from build123d import *

# Parameters (mm, degrees)
F0_R     = 11
F0_R_2   = 11.2
F1_DEPTH = 3.6
F2_R     = 11.2
F2_R_2   = 11
F2_R_3   = 9.7
F3_DEPTH = 1.5
F5_R     = 0.9
F6_DEPTH = 5.1
F7_SIZE  = 1


with BuildPart() as f1:
    # F0 (on Top) → F1 (new body)
    with BuildSketch(Plane.XY):
        with BuildLine():
            ThreePointArc((-2.4878611303, 39.4539370079), (-12.6317197215, 28.3151642022), (-5, 15.3256691841))
            Line((-5, 15.3256691841), (-5, 12.539936204))
            ThreePointArc((-5, 12.539936204), (-11.6913429511, 6.75), (-13.3599033145, -1.9398410831))
            ThreePointArc((-13.3599033145, -1.9398410831), (-11.6913429511, -6.75), (-8.3599033145, -10.6000951209))
            ThreePointArc((-8.3599033145, -10.6000951209), (0, -13.5), (8.3599033145, -10.6000951209))
            ThreePointArc((8.3599033145, -10.6000951209), (11.6913429511, -6.75), (13.3599033145, -1.9398410831))
            ThreePointArc((13.3599033145, -1.9398410831), (11.6913429511, 6.75), (5, 12.539936204))
            Line((5, 12.539936204), (5, 15.3256691841))
            ThreePointArc((5, 15.3256691841), (12.6317197215, 28.3151642022), (2.4878611303, 39.4539370079))
            ThreePointArc((2.4878611303, 39.4539370079), (0, 42.2), (-2.4878611303, 39.4539370079))
        make_face()
        Circle(F0_R, mode=Mode.SUBTRACT)
        with Locations((0, 27)):
            Circle(F0_R_2, mode=Mode.SUBTRACT)
        with BuildLine():
            ThreePointArc((-8.3599033145, -10.6000951209), (-11.6913429511, -6.75), (-13.3599033145, -1.9398410831))
            Line((-13.3599033145, -1.9398410831), (-15.7724188434, -3.3327075731))
            ThreePointArc((-15.7724188434, -3.3327075731), (-30.8375113722, -3.2181919288), (-35.4120422933, -17.572417564))
            ThreePointArc((-35.4120422933, -17.572417564), (-36.5462720397, -21.1), (-32.924181163, -21.8815194439))
            ThreePointArc((-32.924181163, -21.8815194439), (-18.2057916507, -25.0969722734), (-10.7724188434, -11.992961611))
            Line((-10.7724188434, -11.992961611), (-8.3599033145, -10.6000951209))
        make_face()
        with Locations((-23.3826859022, -13.5)):
            Circle(F0_R_2, mode=Mode.SUBTRACT)
        with BuildLine():
            ThreePointArc((13.3599033145, -1.9398410831), (11.6913429511, -6.75), (8.3599033145, -10.6000951209))
            Line((8.3599033145, -10.6000951209), (10.7724188434, -11.992961611))
            ThreePointArc((10.7724188434, -11.992961611), (18.2057916507, -25.0969722734), (32.924181163, -21.8815194439))
            ThreePointArc((32.924181163, -21.8815194439), (36.5462720397, -21.1), (35.4120422933, -17.572417564))
            ThreePointArc((35.4120422933, -17.572417564), (30.8375113722, -3.2181919288), (15.7724188434, -3.3327075731))
            Line((15.7724188434, -3.3327075731), (13.3599033145, -1.9398410831))
        make_face()
        with Locations((23.3826859022, -13.5)):
            Circle(F0_R_2, mode=Mode.SUBTRACT)
    extrude(amount=F1_DEPTH)

    # F2 (on face) → F3 (join)
    with BuildSketch(Plane.XY.offset(3.6)):
        with BuildLine():
            Line((5, 12.539936204), (5, 15.3256691841))
            ThreePointArc((5, 15.3256691841), (12.6317197215, 28.3151642022), (2.4878611303, 39.4539370079))
            ThreePointArc((2.4878611303, 39.4539370079), (0, 42.2), (-2.4878611303, 39.4539370079))
            ThreePointArc((-2.4878611303, 39.4539370079), (-12.6317197215, 28.3151642022), (-5, 15.3256691841))
            Line((-5, 15.3256691841), (-5, 12.539936204))
            ThreePointArc((-5, 12.539936204), (-11.6913429511, 6.75), (-13.3599033145, -1.9398410831))
            Line((-13.3599033145, -1.9398410831), (-15.7724188434, -3.3327075731))
            ThreePointArc((-15.7724188434, -3.3327075731), (-30.8375113722, -3.2181919288), (-35.4120422933, -17.572417564))
            ThreePointArc((-35.4120422933, -17.572417564), (-36.5462720397, -21.1), (-32.924181163, -21.8815194439))
            ThreePointArc((-32.924181163, -21.8815194439), (-18.2057916507, -25.0969722734), (-10.7724188434, -11.992961611))
            Line((-10.7724188434, -11.992961611), (-8.3599033145, -10.6000951209))
            ThreePointArc((-8.3599033145, -10.6000951209), (0, -13.5), (8.3599033145, -10.6000951209))
            Line((8.3599033145, -10.6000951209), (10.7724188434, -11.992961611))
            ThreePointArc((10.7724188434, -11.992961611), (18.2057916507, -25.0969722734), (32.924181163, -21.8815194439))
            ThreePointArc((32.924181163, -21.8815194439), (36.5462720397, -21.1), (35.4120422933, -17.572417564))
            ThreePointArc((35.4120422933, -17.572417564), (30.8375113722, -3.2181919288), (15.7724188434, -3.3327075731))
            Line((15.7724188434, -3.3327075731), (13.3599033145, -1.9398410831))
            ThreePointArc((13.3599033145, -1.9398410831), (11.6913429511, 6.75), (5, 12.539936204))
        make_face()
        with Locations((-23.3826859022, -13.5)):
            Circle(F2_R, mode=Mode.SUBTRACT)
        with Locations((23.3826859022, -13.5)):
            Circle(F2_R, mode=Mode.SUBTRACT)
        Circle(F2_R_2, mode=Mode.SUBTRACT)
        with Locations((0, 27)):
            Circle(F2_R, mode=Mode.SUBTRACT)
        with Locations((0, 27)):
            Circle(F2_R)
        with Locations((0, 27)):
            Circle(F2_R_3, mode=Mode.SUBTRACT)
        with Locations((-23.3826859022, -13.5)):
            Circle(F2_R)
        with Locations((-23.3826859022, -13.5)):
            Circle(F2_R_3, mode=Mode.SUBTRACT)
        with Locations((23.3826859022, -13.5)):
            Circle(F2_R)
        with Locations((23.3826859022, -13.5)):
            Circle(F2_R_3, mode=Mode.SUBTRACT)
        Circle(F2_R_2)
        Circle(F2_R_3, mode=Mode.SUBTRACT)
    extrude(amount=F3_DEPTH)

    # F5 (on face) → F6 (cut, through all)
    with BuildSketch(Plane.XY.offset(5.1)):
        with Locations((0, 39.7)):
            Circle(F5_R)
        with Locations((0, 13.932802694)):
            Circle(F5_R)
        with Locations((-12.0661610789, -6.966401347)):
            Circle(F5_R)
        with Locations((-34.3812085302, -19.85)):
            Circle(F5_R)
        with Locations((12.0661610789, -6.966401347)):
            Circle(F5_R)
        with Locations((34.3812085302, -19.85)):
            Circle(F5_R)
    extrude(amount=-F6_DEPTH, mode=Mode.SUBTRACT)

    # F7
    f7_edges = [f1.edges().sort_by_distance(p)[0] for p in [
        (-18.205792, -25.096972, 5.1),
        (-9.566161, -11.296528, 5.1),
        (0, -13.5, 5.1),
        (9.566161, -11.296528, 5.1),
        (18.205792, -25.096972, 5.1),
        (30.837511, -3.218192, 5.1),
        (14.566161, -2.636274, 5.1),
        (11.691343, 6.75, 5.1),
        (5, 13.932803, 5.1),
        (12.63172, 28.315164, 5.1),
        (-12.63172, 28.315164, 5.1),
        (-5, 13.932803, 5.1),
        (-11.691343, 6.75, 5.1),
        (-14.566161, -2.636274, 5.1),
        (-30.837511, -3.218192, 5.1),
    ]]
    chamfer(f7_edges, length=F7_SIZE)


solid = f1.part
Input: part model. Units: mm. Frame: model coordinates. A direction names the side the tool comes from. Give positions to 0.01 mm unless a question says otherwise; leave off trailing zeros. Loops run counter-clockwise (first coordinate to the right, second up) from the corner with the lowest first, then second, coordinate; pieces in that order, holes last. Notation, with made-up numbers: M 11,54.5 L 55,54.5 A18 cw 55,82.5 Z; hole C -14,50 d2. An arc over 180 degrees is marked long. Use one line per item in the form item = value.
1. Line query: L1, parallel to Y at x = 0, z = 2; L2, parallel to X at y = 39.7, z = 2.25; L3, parallel to Y at x = 0.5, z = 2.1. Output: solid intervals per line, ascending.
Numbers:
L1 = -13.5 to -11, 11 to 13.03, 14.83 to 15.8, 38.2 to 38.8, 40.6 to 42.2
L2 = -2.5 to -0.9, 0.9 to 2.5
L3 = -13.49 to -10.99, 10.99 to 13.18, 14.68 to 15.81, 38.19 to 38.95, 40.45 to 42.15
2. Section query B-B, the plane y = 27. Return the cut outline in (x, z).
Numbers:
outline = M -12.7,0 L -11.2,0 L -11.2,3.6 L -9.7,3.6 L -9.7,5.1 L -11.7,5.1 L -12.7,4.1 Z; M 9.7,3.6 L 11.2,3.6 L 11.2,0 L 12.7,0 L 12.7,4.1 L 11.7,5.1 L 9.7,5.1 Z
3. Section query A-A, the plane x = 0. Count the separate pieces of the cut face and the enclosed holes in it, and give its area (3 significant figures).
Numbers:
separate_pieces = 5
enclosed_holes = 0
area = 47.2 mm²
4. Pull-direction query (Y, two-part tool) for faces 4 (the face through (-0.1, -12.7, 4.9)), 5 (the face through (-11.816, 28.168, 4.926)); classes: released by +Y, released by -Y, zero draft, split by the parting line, or undercut.
Numbers:
face_4 = released by -Y
face_5 = undercut
5. First-contact query: pin 1 (11 mm diameter, centred on x = -3, y = 22.5, fed in from -Z); pin 2 (1.4 mm diameter, centred on y = 14.5, z = 2, fed in from +X); pin 3 (0.8 mm diameter, centred on y = 14.5, z = 1.5, fed in from -X). Flat tips, straight axial feed; report the tip coordinate or a pass-through.
Numbers:
pin_1 = 3.6
pin_2 = 5
pin_3 = -5
6. Reachability of faces 1 (the face through (-35.045, -19.242, 2.586)), 2 (the face through (0, 37, 3.6)), 3 (the face through (5, 14, 2)) from +Z, -Z, +X, -X, +Y, -Y: full face, straight path, thin tool, end or side. Return the list, or none.
Numbers:
face_1 = +Z, -Z
face_2 = -Z
face_3 = +Z, -Z, +X
